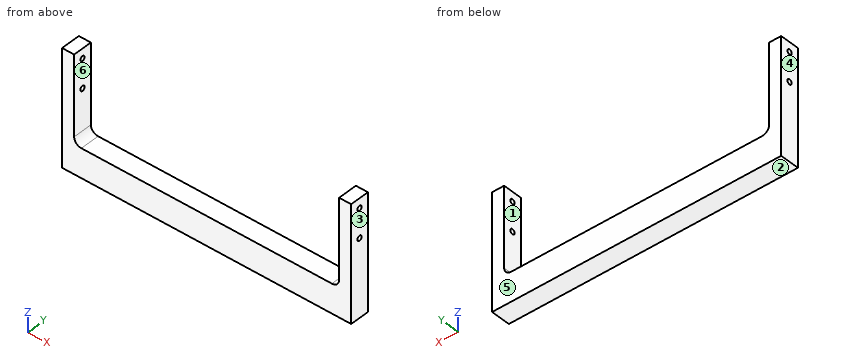
from build123d import *

# Parameters (mm, degrees)
EXTRUDE1_DEPTH               = 25.4
FILLET1_R                    = 9.525
F_5_16_18_TAPPED_HOLE1_D     = 6.5278
F_5_16_18_TAPPED_HOLE1_DEPTH = 15.875
F_5_16_18_TAPPED_HOLE2_D     = 6.5278


with BuildPart() as part:
    # Sketch1 → Extrude1 (new body)
    with BuildSketch(Plane(origin=(0, 0, 0), x_dir=(1, 0, 0), z_dir=(0, 1, 0))):
        Polygon((174.625, -152.4), (190.5, -152.4), (190.5, 0), (-190.5, 0), (-190.5, -152.4), (-174.625, -152.4), (-174.625, -38.1), (174.625, -38.1), align=None)
    extrude(amount=EXTRUDE1_DEPTH)

    # Fillet1
    fillet1_edges = [part.edges().sort_by_distance(p)[0] for p in [
        (174.625, 12.7, 38.1),
        (-174.625, 12.7, 38.1),
    ]]
    fillet(fillet1_edges, radius=FILLET1_R)

    # 5/16-18 Tapped Hole1
    with Locations(Plane(origin=(190.5, 0, 0), x_dir=(0, 0, -1), z_dir=(1, 0, 0))):
        with Locations((-139.7, 12.7), (-101.6, 12.7)):
            Hole(F_5_16_18_TAPPED_HOLE1_D / 2, depth=F_5_16_18_TAPPED_HOLE1_DEPTH)

    # 5/16-18 Tapped Hole2 (through all)
    with Locations(Plane.ZY.offset(190.5)):
        with Locations((101.6, 12.7), (139.7, 12.7)):
            Hole(F_5_16_18_TAPPED_HOLE2_D / 2)


solid = part.part
For this review, take the finished solid that the model builds, in its own axes (mm). Face numbers are marked on the shaded views. A direction names the side the tool comes from. Round coordinates to 2 decimals unless told otherwise and drop trailing zeros. Order: outer loops, then holes, each group sorted by start corner. A loop starts at its lowest first (then second) coordinate and runs counter-clockwise, first axis right, second up. Notation, with made-up numbers: (46.25, -10) -> (94.25, -10) arc R19 ccw to (94.25, 0) -> close; hole circle Ø11 at (41, 73). An arc over 180 degrees is marked (long way). Write item = value, one per line. Start each with the question number.
1) Take a section at C-C on z = 44. State the section outline as (x, y) points.
2) The part is to be moulded in two halves that separate along X. For the marked faces 3, 4, 5 and 6, say which applies: +X half, -X half, draft (parallel to the pull), parting line (faces both ways), or undercut.
3) To check wall thickness, follow line 1 (X direction, y = 11.75, z = 134) (3 decimals); line 2 (Y direction, x = 185, z = 101.6); line 3 (Y direction, x = -182, z = 139). State the ranges of each line that lie inside material, in increasing order. Write a range as from..to.
4) Tool access review of the marked faces 1 and 2: name each direction out of +Z, -Z, +X, -X, +Y, -Y from which nothing blocks a thin tool from reaching the whole face with its end or side.
5) Take a section at A-A on z = 118.5. State the section outline as (x, y) points (3 decimals).
6) Insertion check: pin 1 (5 mm diameter, centred on x = -89, y = 11.5, fed in from +Z); pin 2 (6 mm diameter, centred on y = 12.7, z = 139.7, fed in from -X). Each pin has a flat end and moves straight along its axis. Give the tip position at first contact, or say it passes through.
7) Take a section at D-D on x = 99.5. State the section outline as (y, z) points, plus the area to 3 significant figures.
8) Take a section at B-B on y = 4.75. State the section outline as (x, z) points (3 decimals), plus the area to 3 significant figures.
Verdict:
q1.outline = (-190.5, 0) -> (-173.91, 0) -> (-173.91, 25.4) -> (-190.5, 25.4) -> close; (173.91, 0) -> (190.5, 0) -> (190.5, 25.4) -> (173.91, 25.4) -> close
q2.face_3 = +X half
q2.face_4 = -X half
q2.face_5 = draft
q2.face_6 = undercut
q3.line_1 = -190.5..-174.625, 174.625..190.5
q3.line_2 = 0..9.44, 15.96..25.4
q3.line_3 = 0..9.51, 15.89..25.4
q4.face_1 = +Z, +Y, -Y
q4.face_2 = -Z, +X, -X, +Y, -Y
q5.outline = (-190.5, 0) -> (-174.625, 0) -> (-174.625, 25.4) -> (-190.5, 25.4) -> close; (174.625, 0) -> (190.5, 0) -> (190.5, 25.4) -> (174.625, 25.4) -> close
q6.pin_1 = 38.1
q6.pin_2 = through
q7.outline = (0, 0) -> (25.4, 0) -> (25.4, 38.1) -> (0, 38.1) -> close
q7.area = 968 mm2
q8.outline = (-190.5, 0) -> (190.5, 0) -> (190.5, 152.4) -> (174.625, 152.4) -> (174.625, 47.625) arc R9.525 cw to (165.1, 38.1) -> (-165.1, 38.1) arc R9.525 cw to (-174.625, 47.625) -> (-174.625, 152.4) -> (-190.5, 152.4) -> close
q8.area = 18,200 mm2
